from build123d import *

# Parameters (mm, degrees)
SKETCH1_R           = 11.5
BOSS_EXTRUDE5_DEPTH = 2
SKETCH4_R           = 5
BOSS_EXTRUDE6_DEPTH = 8
CUT_EXTRUDE2_DEPTH  = 0.5
FILLET1_R           = 0.5


with BuildPart() as part:
    # Sketch1 → Boss-Extrude5 (new body)
    with BuildSketch(Plane(origin=(0, 0, 0), x_dir=(1, 0, 0), z_dir=(0, 1, 0))):
        with Locations(Location((-5.408676197, -40.3067379, 0), (0, 0, 270))):
            Circle(SKETCH1_R)
    extrude(amount=BOSS_EXTRUDE5_DEPTH)

    # Sketch4 → Boss-Extrude6 (add)
    with BuildSketch(Plane(origin=(0, 2, 0), x_dir=(1, 0, 0), z_dir=(0, 1, 0))):
        with Locations(Location((-5.408676197, -40.3067379, 0), (0, 0, 270))):
            Circle(SKETCH4_R)
    extrude(amount=BOSS_EXTRUDE6_DEPTH)

    # Sketch5 → Cut-Extrude2 (cut)
    # profile 1 of 2: a face of its own
    with BuildSketch(Plane.XZ):
        Polygon((-11.816511362, 36.397340578), (-9.664612628, 36.397340578), (-9.664612628, 44.372024123), (-12.069675919, 43.865695009), (-12.069675919, 44.878353237), (-9.644834147, 45.38468235), (-8.272207565, 45.38468235), (-8.272207565, 36.397340578), (-6.120308831, 36.397340578), (-6.120308831, 35.38468235), (-11.816511362, 35.38468235), align=None)
    # profile 2 of 2: a face of its own
    with BuildSketch(Plane.XZ):
        with BuildLine():
            add(Edge.make_bspline(
                [(-0.550688578, 45.637846907), (-0.415938804, 45.633730166), (-0.152802852, 45.625691098), (0.229163714, 45.561237383), (0.586683797, 45.456245103), (0.920332152, 45.309789042), (1.227359965, 45.117028679), (1.510292763, 44.884079449), (1.767374377, 44.607527173), (1.998267531, 44.289408333), (2.204159406, 43.931981409), (2.381194089, 43.535679405), (2.534314002, 43.103516508), (2.654820834, 42.631767759), (2.752456274, 42.123354369), (2.816869131, 41.576005545), (2.859979178, 40.99125567), (2.864632597, 40.588485261), (2.867032941, 40.380726654)],
                knots=[0, 0, 0, 0, 0.914621173, 1.786049105, 2.621809963, 3.439570598, 4.25200759, 5.075726843, 5.921440778, 6.808834034, 7.739519474, 8.717306742, 9.75236949, 10.849108534, 12.020406428, 13.265380358, 14.589417808, 16, 16, 16, 16], degree=3))
            add(Edge.make_bspline(
                [(2.867032941, 40.380726654), (2.864644222, 40.173625568), (2.86001379, 39.772168798), (2.816709133, 39.188761145), (2.752698639, 38.642668217), (2.654549419, 38.135010363), (2.534332528, 37.663871958), (2.381219253, 37.231685314), (2.204051011, 36.835485659), (1.998914362, 36.478161083), (1.766700275, 36.161674678), (1.510372243, 35.885227112), (1.227339233, 35.652351187), (0.92033771, 35.459571593), (0.58668227, 35.313120715), (0.229164144, 35.208127003), (-0.152802968, 35.143673687), (-0.415938843, 35.135634563), (-0.550688578, 35.131517794)],
                knots=[0, 0, 0, 0, 1.407597425, 2.728568576, 3.974862697, 5.143000578, 6.240902623, 7.277062968, 8.255887098, 9.187559452, 10.072280029, 10.918890773, 11.743483511, 12.556782025, 13.375409826, 14.212056939, 15.084408948, 16, 16, 16, 16], degree=3))
            add(Edge.make_bspline(
                [(-0.550688578, 35.131517794), (-0.6854385, 35.135634386), (-0.948574743, 35.143673163), (-1.330539237, 35.208128951), (-1.688066752, 35.313113795), (-2.021688201, 35.459596777), (-2.328815845, 35.652257252), (-2.611716883, 35.885875244), (-2.870168983, 36.160946148), (-3.102194243, 36.478253797), (-3.307287706, 36.835508053), (-3.48508341, 37.231281228), (-3.635082086, 37.66432144), (-3.756126667, 38.134940569), (-3.854016818, 38.642688789), (-3.91810349, 39.188755145), (-3.961386204, 39.772170452), (-3.966019764, 40.173626131), (-3.968410097, 40.380726654)],
                knots=[0, 0, 0, 0, 0.915500487, 1.787766207, 2.624330562, 3.442877389, 4.256095455, 5.080606629, 5.930200102, 6.814833167, 7.746413364, 8.725140674, 9.759714696, 10.857508142, 12.025530477, 13.27170132, 14.592541807, 16, 16, 16, 16], degree=3))
            add(Edge.make_bspline(
                [(-3.968410097, 40.380726654), (-3.966008131, 40.588484695), (-3.961351569, 40.991254008), (-3.918263552, 41.576011567), (-3.853774368, 42.123333768), (-3.756398925, 42.631837847), (-3.63506368, 43.103067057), (-3.485058278, 43.536083527), (-3.307396088, 43.931958995), (-3.101547546, 44.289315613), (-2.870846186, 44.608258357), (-2.611637461, 44.883431398), (-2.32883653, 45.117122569), (-2.021682655, 45.30976387), (-1.688068275, 45.45625202), (-1.330538808, 45.561235436), (-0.948574858, 45.625691622), (-0.685438539, 45.633730344), (-0.550688578, 45.637846907)],
                knots=[0, 0, 0, 0, 1.410442812, 2.734349433, 3.979200347, 5.150382505, 6.24701318, 7.280491394, 8.258182046, 9.188775525, 10.076081097, 10.924774691, 11.748412552, 12.560769267, 13.378449099, 14.214127375, 15.085469201, 16, 16, 16, 16], degree=3))
        make_face()
        with BuildLine():
            add(Edge.make_bspline(
                [(-0.554644274, 44.62518868), (-0.635989574, 44.622401752), (-0.795646719, 44.616931825), (-1.026841529, 44.566459489), (-1.242386869, 44.482103579), (-1.441486777, 44.363897306), (-1.625737076, 44.213545447), (-1.792639211, 44.028975958), (-1.943217724, 43.811177792), (-2.076899469, 43.560448999), (-2.195580983, 43.277641024), (-2.297639092, 42.961856636), (-2.383967094, 42.612798562), (-2.454448483, 42.230321244), (-2.509050303, 41.815044266), (-2.548039786, 41.366310053), (-2.571798824, 40.8846772), (-2.574574099, 40.552168459), (-2.576005033, 40.380726654)],
                knots=[0, 0, 0, 0, 0.748569641, 1.469224287, 2.167313872, 2.872447611, 3.593306944, 4.349889458, 5.156880845, 6.026416454, 6.962619852, 7.978571635, 9.080333099, 10.272657594, 11.559295133, 12.937179704, 14.420807114, 16, 16, 16, 16], degree=3))
            add(Edge.make_bspline(
                [(-2.576005033, 40.380726654), (-2.574582635, 40.209943239), (-2.571824242, 39.878750606), (-2.547925246, 39.398448218), (-2.509225008, 38.951001137), (-2.45425411, 38.536431355), (-2.383976272, 38.154591028), (-2.297666503, 37.805513593), (-2.195476658, 37.489802584), (-2.077472273, 37.20728493), (-1.942625912, 36.957849971), (-1.792702591, 36.740354541), (-1.625721415, 36.555827706), (-1.441490789, 36.40546523), (-1.242385817, 36.287261689), (-1.026841818, 36.202905056), (-0.795646642, 36.152432918), (-0.635989549, 36.146962963), (-0.554644274, 36.144176021)],
                knots=[0, 0, 0, 0, 1.575434164, 3.05516895, 4.435080037, 5.717581461, 6.91165956, 8.015041434, 9.032487421, 9.970067734, 10.835534704, 11.643712969, 12.401408222, 13.123327754, 13.829498565, 14.528614861, 15.250329405, 16, 16, 16, 16], degree=3))
            add(Edge.make_bspline(
                [(-0.554644274, 36.144176021), (-0.472616683, 36.146871841), (-0.312254594, 36.152142109), (-0.0794757, 36.203726771), (0.138133244, 36.286201975), (0.338090945, 36.405582767), (0.522379645, 36.55579412), (0.689341824, 36.740364859), (0.839280394, 36.957844948), (0.974082065, 37.207294623), (1.092268814, 37.489765126), (1.193740002, 37.805824707), (1.283313605, 38.15424386), (1.352654751, 38.536487567), (1.407914192, 38.950984355), (1.446528422, 39.398453194), (1.470452529, 39.878749229), (1.473207332, 40.20994277), (1.474627878, 40.380726654)],
                knots=[0, 0, 0, 0, 0.75484838, 1.475711535, 2.185326637, 2.890664395, 3.611732298, 4.368533717, 5.175758594, 6.040204595, 6.976678868, 7.992924601, 9.096493949, 10.289163424, 11.570151914, 12.948435155, 14.426424335, 16, 16, 16, 16], degree=3))
            add(Edge.make_bspline(
                [(1.474627878, 40.380726654), (1.473198806, 40.55216893), (1.470427142, 40.884678585), (1.446642874, 41.366305056), (1.407739604, 41.815061077), (1.352847963, 42.230264739), (1.28330429, 42.6131457), (1.193712582, 42.961545506), (1.092373097, 43.277678471), (0.973509023, 43.560439245), (0.839872237, 43.811182841), (0.689278446, 44.028965642), (0.522395306, 44.213579032), (0.338086936, 44.363779771), (0.138134314, 44.483163303), (-0.079475991, 44.565637773), (-0.312254517, 44.617222634), (-0.472616657, 44.622492874), (-0.554644274, 44.62518868)],
                knots=[0, 0, 0, 0, 1.577332685, 3.059212465, 4.435473965, 5.720595916, 6.91151592, 8.013466492, 9.028221541, 9.963322143, 10.831833488, 11.637874284, 12.393565586, 13.113575787, 13.817878918, 14.526453118, 15.246258873, 16, 16, 16, 16], degree=3))
        make_face(mode=Mode.SUBTRACT)
    extrude(amount=-CUT_EXTRUDE2_DEPTH, mode=Mode.SUBTRACT)

    # Fillet1
    fillet1_edges = [part.edges().sort_by_distance(p)[0] for p in [
        (-5.408676197, 0, 28.8067379),
        (-5.408676197, 2, 28.8067379),
    ]]
    fillet(fillet1_edges, radius=FILLET1_R)


solid = part.part
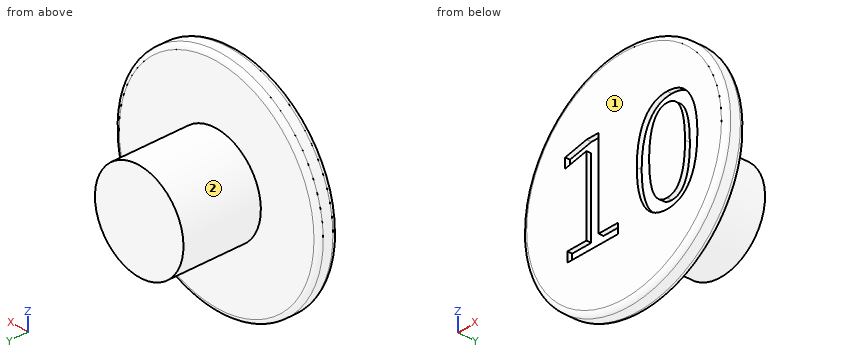
Here's how the part is built. I have some questions about the finished solid (model axes, mm). Face numbers are marked on the shaded views. A direction names the side the tool comes from. Give positions to 0.01 mm unless a question says otherwise; leave off trailing zeros. Order: outer loops, then holes, each group sorted by start corner. A loop starts at its lowest first (then second) coordinate and runs counter-clockwise, first axis right, second up. Notation, with made-up numbers: M 12.5,33 L 24.5,33 A30 ccw 24.5,63 Z; hole C 5,-19.75 d9. An arc over 180 degrees is marked long. Answer as a JSON object with one key per item and string values. Group by question number.
1) On a 3-axis mill with a long thin cutter (end or side, diameter ignored), from which of +Z, -Z, +X, -X, +Y, -Y can I reach the whole of each face in a straight line? I mean the marked faces 1 and 2. Say none if no direction works.
2) Please list where these lines run through material, in increasing order: L1, parallel to Y at x = -1.25, z = 50.5; L2, parallel to Z at x = -5.5, y = 1; L3, parallel to Y at x = 0.75, z = 44. Write a range as [from, to].
3) I'm going to push flat-ended pins straight in: pin 1 Ø0.6 at (x, y) = (-7, 0) entering from -Z; pin 2 Ø0.6 at (y, z) = (0, 44.5) entering from +X; pin 3 Ø0.6 at (x, y) = (-9, 0) entering from -Z. Where does each tip first touch, or does it pass through?
4) Suppose I cut it at A-A, the plane y = 9.5. Write out the boundary of the cut face in (x, z).
Results found:
{
 "1": {"face 1": "+Z, -Z, +X, -X, -Y", "face 2": "+Y"},
 "2": {"L1": "[0, 2]", "L2": "[28.81, 51.81]", "L3": "[0.5, 2]"},
 "3": {"pin 1": "z = 28.95", "pin 2": "x = 5.29", "pin 3": "z = 29.4"},
 "4": {"outline": "C -5.41,40.31 d10"}
}
